The listing builds one solid part. Answer for the finished solid, in the listing's coordinates (mm). Face numbers are marked on the shaded views. Coordinates: 2 decimals unless noted, no trailing zeros. Write each loop counter-clockwise with the first axis right and the second up, starting at its lowest first coordinate (ties: lowest second). Pieces come first, ordered by that corner, then holes.
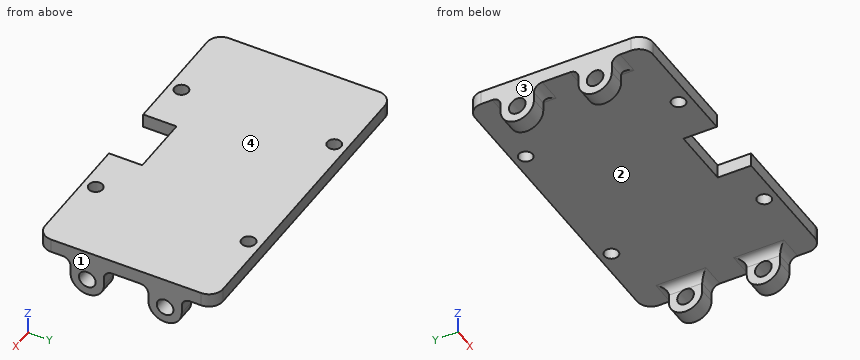
from build123d import *

# Parameters (mm, degrees)
SKETCH_1_R      = 1.25
EXTRUDE_1_DEPTH = 2.5
SKETCH_3_R      = 1.5
EXTRUDE_2_DEPTH = 3
EXTRUDE_START   = -3
SKETCH_4_R      = 1.5
EXTRUDE_3_DEPTH = 3
FILLET_1_R      = 1.5
FILLET_2_R      = 2.5


with BuildPart() as part:
    # 草图1 → 凸台-拉伸1 (new body)
    with BuildSketch(Plane.XY):
        Polygon((-28.5, -16), (-16, -16), (-5.5, -16), (-5.5, -10), (0, -10), (5.5, -10), (5.5, -16), (16, -16), (28.5, -16), (28.5, 16), (16, 16), (-16, 16), (-28.5, 16), align=None)
        with Locations((-13.75, -13.75)):
            Circle(SKETCH_1_R, mode=Mode.SUBTRACT)
        with Locations((13.75, -13.75)):
            Circle(SKETCH_1_R, mode=Mode.SUBTRACT)
        with Locations((-13.75, 13.75)):
            Circle(SKETCH_1_R, mode=Mode.SUBTRACT)
        with Locations((13.75, 13.75)):
            Circle(SKETCH_1_R, mode=Mode.SUBTRACT)
    extrude(amount=EXTRUDE_1_DEPTH)

    # 草图3 → 凸台-拉伸2 (add)
    # profile 1 of 2: a face of its own
    with BuildSketch(Plane.ZY.offset(28.5)):
        with BuildLine():
            Line((-3, 4), (0, 4))
            Line((0, 4), (0, 10))
            Line((0, 10), (-3, 10))
            ThreePointArc((-3, 10), (-6, 7), (-3, 4))
        make_face()
        with Locations((-3, 7)):
            Circle(SKETCH_3_R, mode=Mode.SUBTRACT)
    # profile 2 of 2: a face of its own
    with BuildSketch(Plane.ZY.offset(28.5)):
        with BuildLine():
            Line((-3, -4), (0, -4))
            Line((0, -4), (0, -10))
            Line((0, -10), (-3, -10))
            ThreePointArc((-3, -10), (-6, -7), (-3, -4))
        make_face()
        with Locations((-3, -7)):
            Circle(SKETCH_3_R, mode=Mode.SUBTRACT)
    extrude(amount=-EXTRUDE_2_DEPTH)

    # 草图4 → 凸台-拉伸3 (add)
    # profile 1 of 2: a face of its own
    with BuildSketch(Plane(origin=(28.5, 0, 0), x_dir=(0, 0, -1), z_dir=(1, 0, 0)).offset(EXTRUDE_START)):
        with BuildLine():
            Line((3, -4), (0, -4))
            Line((0, -4), (0, -10))
            Line((0, -10), (3, -10))
            ThreePointArc((3, -10), (6, -7), (3, -4))
        make_face()
        with Locations(Location((3, -7, 0), (0, 0, 180))):
            Circle(SKETCH_4_R, mode=Mode.SUBTRACT)
    # profile 2 of 2: a face of its own
    with BuildSketch(Plane(origin=(28.5, 0, 0), x_dir=(0, 0, -1), z_dir=(1, 0, 0)).offset(EXTRUDE_START)):
        with BuildLine():
            Line((3, 10), (0, 10))
            Line((0, 10), (0, 4))
            Line((0, 4), (3, 4))
            ThreePointArc((3, 4), (6, 7), (3, 10))
        make_face()
        with Locations(Location((3, 7, 0), (0, 0, 180))):
            Circle(SKETCH_4_R, mode=Mode.SUBTRACT)
    extrude(amount=EXTRUDE_3_DEPTH)

    # 圆角1
    fillet_1_edges = [part.edges().sort_by_distance(p)[0] for p in [
        (-25.5, 7, 0),
        (-27, 10, 0),
        (-27, 4, 0),
        (-25.5, -7, 0),
        (-27, -4, 0),
        (-27, -10, 0),
        (25.5, -7, 0),
        (27, -10, 0),
        (27, -4, 0),
        (25.5, 7, 0),
        (27, 4, 0),
        (27, 10, 0),
    ]]
    fillet(fillet_1_edges, radius=FILLET_1_R - 0.0001)  # a hair under: the kernel refuses the full size

    # 圆角2
    fillet_2_edges = [part.edges().sort_by_distance(p)[0] for p in [
        (-28.5, -16, 1.25),
        (-28.5, 16, 1.25),
        (28.5, 16, 1.25),
        (28.5, -16, 1.25),
    ]]
    fillet(fillet_2_edges, radius=FILLET_2_R)


solid = part.part
Q1. The part is cut by section C-C, the plane z = 1. Write down the section's boundary in (x, y), then the cut area to 3 significant figures.
Answers below:
outline: (-28.5, -13.5) arc R2.5 ccw to (-26, -16) - (-5.5, -16) - (-5.5, -10) - (5.5, -10) - (5.5, -16) - (26, -16) arc R2.5 ccw to (28.5, -13.5) - (28.5, 13.5) arc R2.5 ccw to (26, 16) - (-26, 16) arc R2.5 ccw to (-28.5, 13.5) - close; hole circle Ø2.5 at (-13.75, -13.75); hole circle Ø2.5 at (-13.75, 13.75); hole circle Ø2.5 at (13.75, -13.75); hole circle Ø2.5 at (13.75, 13.75)
area: 1,730 mm2
Q2. The part is cut by section B-B, the plane y = 7. State how many separate pieces and enclosed holes the cut face has, then the cut area to 3 significant figures.
Answers below:
separate pieces: 3
enclosed holes: 0
area: 161 mm2
Q3. The part is cut by section D-D, the plane x = -22. Write down the section's boundary in (y, z), then the cut area to 3 significant figures.
Answers below:
outline: (-16, 0) - (16, 0) - (16, 2.5) - (-16, 2.5) - close
area: 80.0 mm2
Q4. The part is cut by section A-A, the plane x = -13.75. Write down the section's boundary in (y, z), then the cut area to 3 significant figures.
Answers below:
outline: (-16, 0) - (-15, 0) - (-15, 2.5) - (-16, 2.5) - close; (-12.5, 0) - (12.5, 0) - (12.5, 2.5) - (-12.5, 2.5) - close; (15, 0) - (16, 0) - (16, 2.5) - (15, 2.5) - close
area: 67.5 mm2
Q5. Find the intervals of material crossed by probe 1 along Y at (x, z) = (-13.75, 1.25); probe 2 along Y at (x, z) = (-27.1, -3); probe 3 along X at (y, z) = (8, -5), in increasing order.
Answers below:
probe 1: y = -16 to -15, -12.5 to 12.5, 15 to 16
probe 2: y = -10 to -8.5, -5.5 to -4, 4 to 5.5, 8.5 to 10
probe 3: x = -28.5 to -25.5, 25.5 to 28.5
Q6. Given pin 1 (0.8 mm diameter, centred on x = 0, z = 1.5, fed in from -Y); pin 2 (1.7 mm diameter, centred on x = 27.5, z = -2.5, fed in from +Y); pin 3 (10 mm diameter, centred on x = 9, y = 8.5, fed in from -Z), each flat-ended and moving along its own axis, determine where each tip first touches the part or whether it passes through.
Answers below:
pin 1: stops at y = -10
pin 2: stops at y = 10
pin 3: stops at z = 0
Q7. Determine the mould class of the marked faces 1, 2, 3 and 4 for opening direction X: released by +X, released by -X, zero draft, split by the parting line, or undercut.
Answers below:
face 1: released by +X
face 2: undercut
face 3: released by -X
face 4: zero draft
